from build123d import *

# Parameters (mm, degrees)
F1_DEPTH = 2.286
F3_DEPTH = 23.495
F5_DEPTH = 12.7
F6_R     = 6.604
F7_DEPTH = 1.905
F9_DEPTH = 17.25


with BuildPart() as f1:
    # F0 (on Top) → F1 (new body)
    with BuildSketch(Plane.XY):
        with BuildLine():
            ThreePointArc((4.8862001852, 0), (6.4854349991, 2.3194773824), (7.0485, 5.08))
            ThreePointArc((7.0485, 5.08), (-2.7605226176, 11.5654349991), (-4.8862001852, 0))
            ThreePointArc((-4.8862001852, 0), (0, 1.9685), (4.8862001852, 0))
        make_face()
        with BuildLine():
            ThreePointArc((4.8862001852, 0), (0, 1.9685), (-4.8862001852, 0))
            ThreePointArc((-4.8862001852, 0), (0, -1.9685), (4.8862001852, 0))
        make_face()
        with BuildLine():
            ThreePointArc((4.8862001852, 0), (0, -1.9685), (-4.8862001852, 0))
            ThreePointArc((-4.8862001852, 0), (-2.7605226176, -11.5654349991), (7.0485, -5.08))
            ThreePointArc((7.0485, -5.08), (6.4854349991, -2.3194773824), (4.8862001852, 0))
        make_face()
    extrude(amount=F1_DEPTH)

    # F2 (on face) → F3 (join)
    with BuildSketch(Plane(origin=(0, 0, 0), x_dir=(1, 0, 0), z_dir=(0, 0, -1))):
        with BuildLine():
            ThreePointArc((4.2197649224, 0), (5.9783000739, 2.2741589093), (6.604, 5.08))
            ThreePointArc((6.604, 5.08), (-2.8058410907, 11.0583000739), (-4.2197649224, 0))
            ThreePointArc((-4.2197649224, 0), (0, 1.524), (4.2197649224, 0))
        make_face()
        with BuildLine():
            ThreePointArc((4.2197649224, 0), (0, 1.524), (-4.2197649224, 0))
            ThreePointArc((-4.2197649224, 0), (0, -1.524), (4.2197649224, 0))
        make_face()
        with BuildLine():
            ThreePointArc((4.2197649224, 0), (0, -1.524), (-4.2197649224, 0))
            ThreePointArc((-4.2197649224, 0), (-2.8058410907, -11.0583000739), (6.604, -5.08))
            ThreePointArc((6.604, -5.08), (5.9783000739, -2.2741589093), (4.2197649224, 0))
        make_face()
    extrude(amount=F3_DEPTH)

    # F4 (on face) → F5 (cut)
    with BuildSketch(Plane.XY.offset(2.286)):
        Polygon((1.1175982522, -2.7082355227), (-1.0746682528, -2.7082355227), (-1.0746682528, -10.1121831685), (2.3251036182, -10.1121831685), (2.3251036182, -7.996769622), (1.1162960436, -7.996769622), align=None)
    extrude(amount=-F5_DEPTH, mode=Mode.SUBTRACT)

    # F6 (on face) → F7 (join)
    with BuildSketch(Plane(origin=(0, 0, -23.495), x_dir=(1, 0, 0), z_dir=(0, 0, -1))):
        with Locations((0, 5.08)):
            Circle(F6_R)
    extrude(amount=F7_DEPTH)

    # F8 (on face) → F9 (join)
    with BuildSketch(Plane(origin=(0, 0, -23.495), x_dir=(1, 0, 0), z_dir=(0, 0, -1))):
        with BuildLine():
            ThreePointArc((-5.7929773658, 1.2513933032), (-6.4591589625, 0.142315863), (-6.0144739499, -1.0726351351))
            ThreePointArc((-6.0144739499, -1.0726351351), (-1.0745990182, -3.4566300699), (4.302, -2.3712825742))
            Line((4.302, -2.3712825742), (0, 5.08))
            Line((0, 5.08), (-5.7929773658, 1.2513933032))
        make_face()
    extrude(amount=-F9_DEPTH)


solid = f1.part
Can you work these out from the model? Positions are in its coordinate system, mm. A direction names the side the tool comes from. Round coordinates to 2 decimals unless told otherwise and drop trailing zeros. Loops run counter-clockwise (first coordinate to the right, second up) from the corner with the lowest first, then second, coordinate; pieces in that order, holes last. Notation, with made-up numbers: (-18, 18) - (6, 18) arc R17 ccw to (6, 22) - close; hole circle Ø9 at (-17.5, 41.25). An arc over 180 degrees is marked (long way). Use CSV: the item, a comma, the result in double quotes. Start each with the question number.
1) We'd pull the mould along X, two halves only. Please class faces 1 (the flat face through (0, 5, -23.495)), 2 (the cylindrical face through (-6.457, -0.161, -14.991)), 3 (the flat face through (0, -2.708, -2)): released by +X, released by -X, zero draft, split by the parting line, or undercut.
2) If we section it at C-C on x = 2: Write out the boundary of the cut face in (y, z) (3 decimals), plus the area to 3 significant figures.
3) Please list where these lines run through material, in increasing order: probe 1 along X at (y, z) = (-5.25, -2.75); probe 2 along Z at (x, y) = (-3.5, 4) (3 decimals); probe 3 along Z at (x, y) = (5.75, 1.75). Write a range as [from, to].
4) If we section it at A-A on z = -2.25: Write out the boundary of the cut face in (x, y).
5) For faces 4 (the flat face through (0, 0, 2.286)), 5 (the flat face through (1, -10.112, -4)), 6 (the flat face through (-6, 0, -6.245)), which set-ups out of +Z, -Z, +X, -X, +Y, -Y let a thin tool reach every point of the face, with its end or its side?
6) For pin 1 Ø2 at (x, z) = (1.5, -7.5) entering from +Y; pin 2 Ø1.3 at (x, z) = (1.5, -3.5) entering from -Y; pin 3 Ø1.1 at (y, z) = (-8.5, -3.5) entering from -X, each with a flat end and sliding along its axis, tell me the tip position at first contact or that it passes through.
7) If we section it at D-D on x = -2.5: Write out the boundary of the cut face in (y, z) (3 decimals).
8) If we section it at B-B on z = -16.25: Write out the boundary of the cut face in (x, y).
Geometry results:
1,face 1,"zero draft"
1,face 2,"released by -X"
1,face 3,"undercut"
2,outline,"(-11.839, 0) - (-11.374, 0) - (-11.374, -25.4) - (1.214, -25.4) - (1.214, -23.495) - (11.374, -23.495) - (11.374, 0) - (11.839, 0) - (11.839, 2.286) - (-7.997, 2.286) - (-7.997, -10.414) - (-10.112, -10.414) - (-10.112, 2.286) - (-11.839, 2.286) - close"
2,area,"586 mm2"
3,probe 1,"x = [-6.6, -1.07], [1.12, 6.6]"
3,probe 2,"z = [-23.495, 2.286]"
3,probe 3,"z = [0, 2.29]"
4,outline,"(-4.22, 0) arc R6.6 ccw (long way) to (4.22, 0) arc R6.6 ccw (long way) to start; hole (-1.07, -10.11) - (2.33, -10.11) - (2.33, -8) - (1.12, -8) - (1.12, -2.71) - (-1.07, -2.71) - close"
5,face 4,"+Z, +X, -X, +Y, -Y"
5,face 5,"+Z"
5,face 6,"-X"
6,pin 1,"stops at y = 11.67"
6,pin 2,"stops at y = -11.63"
6,pin 3,"stops at x = -5.95"
7,outline,"(-11.67, 0) - (-11.193, 0) - (-11.193, -25.4) - (1.033, -25.4) - (1.033, -23.495) - (11.193, -23.495) - (11.193, 0) - (11.67, 0) - (11.67, 2.286) - (-11.67, 2.286) - close"
8,outline,"(-6.01, 1.07) arc R1.5 ccw to (-5.79, -1.25) - (-5.51, -1.44) arc R6.6 ccw (long way) to (4.22, 0) arc R6.6 ccw (long way) to (-5.55, 1.5) arc R8.6 ccw to start"
